Read the model definition and answer for the solid it produces. Units are mm, in the model's axes. A direction names the side the tool comes from. Round coordinates to 2 decimals unless told otherwise and drop trailing zeros. Write each loop counter-clockwise with the first axis right and the second up, starting at its lowest first coordinate (ties: lowest second). Pieces come first, ordered by that corner, then holes.
from build123d import *
from build123d.topology import SkipClean

# Parameters (mm, degrees)
SKETCH_2_R          = 9.25
SKETCH_2_R_2        = 7.25
F_19MM_DEPTH        = 19
EXTRUDE_START       = -11
EXTRUDE_7_DEPTH     = 11
SKETCH_630_W        = 27.57
SKETCH_630_H        = 12
EXTRUDE_682_DEPTH   = 14
SKETCH_6_W          = 25.57
SKETCH_6_H          = 10
CUT_EXTRUDE_1_DEPTH = 12
FILLET_1_R          = 5
SKETCH_10_W         = 27.57
SKETCH_10_H         = 1
EXTRUDE_3_DEPTH     = 8


with BuildPart() as part:
    # 草圖2 → 19mm (new body)
    with BuildSketch(Plane(origin=(0, 0, 0), x_dir=(1, 0, 0), z_dir=(0, 1, 0))):
        Circle(SKETCH_2_R)
        Circle(SKETCH_2_R_2, mode=Mode.SUBTRACT)
    extrude(amount=F_19MM_DEPTH)

    # 草圖14 → 伸長-薄件7 (add)
    with SkipClean():  # the faces are left unmerged after this step: merging them gives an invalid solid
        with BuildSketch(Plane(origin=(0, 0, 0), x_dir=(1, 0, 0), z_dir=(0, 1, 0)).offset(EXTRUDE_START)):
            with BuildLine():
                ThreePointArc((7.25, 0), (0, 7.25), (-7.25, 0))
                Line((-7.25, 0), (-9.25, 0))
                ThreePointArc((-9.25, 0), (0, 9.25), (9.25, 0))
                Line((9.25, 0), (7.25, 0))
            make_face()
        extrude(amount=EXTRUDE_7_DEPTH)

    # Sketch 630 → Extrude 682 (add)
    with SkipClean():  # the faces are left unmerged after this step: merging them gives an invalid solid
        with BuildSketch(Plane.XY):
            with Locations((0, -6)):
                Rectangle(SKETCH_630_W, SKETCH_630_H)
        extrude(amount=EXTRUDE_682_DEPTH)

    # 草圖6 → 除料-伸長1 (cut)
    with SkipClean():  # the faces are left unmerged after this step: merging them gives an invalid solid
        with BuildSketch(Plane.XY.offset(14)):
            with Locations((0, -6)):
                Rectangle(SKETCH_6_W, SKETCH_6_H)
        extrude(amount=-CUT_EXTRUDE_1_DEPTH, mode=Mode.SUBTRACT)

    # 圓角1
    # the kernel refuses this fillet: 5 mm, written as the material it takes off along each edge
    with BuildSketch(Plane(origin=(-19.75, 0, 0), x_dir=(0, -1, 0), z_dir=(1, 0, 0))) as fillet_1_piece_1_section:
        with BuildLine():
            CenterArc((FILLET_1_R, -FILLET_1_R), FILLET_1_R, 90, 90)
            Line((0, -FILLET_1_R), (0, 0))
            Line((0, 0), (FILLET_1_R, 0))
        make_face()
    fillet_1_piece_1 = extrude(amount=39.5, mode=Mode.PRIVATE)
    fillet_1_piece_1 = fillet_1_piece_1 & Plane(origin=(0, -1.958227167, 0), x_dir=(1, 0, 0), z_dir=(0, -1, 0)) * Cylinder(7.25, 99, mode=Mode.PRIVATE)
    add(fillet_1_piece_1, mode=Mode.SUBTRACT)

    # 草圖10 → 填料-伸長3 (add)
    with BuildSketch(Plane.XZ.offset(12)):
        with Locations((0, 0.5)):
            Rectangle(SKETCH_10_W, SKETCH_10_H)
    extrude(amount=EXTRUDE_3_DEPTH)


solid = part.part
Q1. Flat-ended cylindrical pins translate along their axes: pin 1 Ø6.5 at (x, z) = (-0.5, 8.5) entering from -Y; pin 2 Ø1.5 at (y, z) = (-7.5, -7) entering from +X; pin 3 Ø6 at (x, z) = (-1, 4) entering from +Y. Find the tip coordinate at first contact, or state that the pin passes through.
Verdict:
pin 1: stops at y = -12
pin 2: stops at x = 6.82
pin 3: stops at y = 0
Q2. Determine the mould class of faces 1 (the flat face through (0, 0, 10)), 2 (the flat face through (0, -6, 2)), 3 (the cylindrical face through (-0.94, 7.12, -7.19)) for opening direction Y: pulls with the +Y half, pulls with the -Y half, needs draft (parallel to the pull), parting line crosses it, or undercut.
Verdict:
face 1: pulls with the +Y half
face 2: undercut
face 3: needs draft
Q3. Which of the six approach directions +Z, -Z, +X, -X, +Y, -Y give full straight-line access (tool end or side, diameter ignored) to faces 4 (the flat face through (0, -11, 8)), 5 (the flat face through (0, -12, 7)), 6 (the cylindrical face through (-0.098, -0.264, 3.398)), 7 (the flat face through (-0.6, -11, -7.4))?
Verdict:
face 4: +Z
face 5: +Z, +X, -X, -Y
face 6: +Y
face 7: -Z, +X, -X, -Y
Q4. Straight lines are drawn through the part: probe 1 along X at (y, z) = (10.5, 0); probe 2 along X at (y, z) = (-3, 13) (3 decimals); probe 3 along Y at (x, z) = (2.5, 11). For each, find the intervals that lie inside material, in ascending order.
Verdict:
probe 1: x = -9.25 to -7.25, 7.25 to 9.25
probe 2: x = -13.785 to -12.785, 12.785 to 13.785
probe 3: y = -12 to -11, -1 to 0
Q5. Section D-D (x = 11.75) is taken. Determine the outline of the cut face in (y, z).
Verdict:
outline: (-20, 0) - (0, 0) - (0, 14) - (-1, 14) - (-1, 2) - (-11, 2) - (-11, 14) - (-12, 14) - (-12, 1) - (-20, 1) - close
Q6. Section B-B (y = -7.5) is taken. Determine the outline of the cut face in (x, z) (3 decimals).
Verdict:
outline: (-13.785, 0) - (-9.25, 0) arc R9.25 ccw to (9.25, 0) - (13.785, 0) - (13.785, 14) - (12.785, 14) - (12.785, 2) - (-12.785, 2) - (-12.785, 14) - (-13.785, 14) - close; hole (-7.25, 0) arc R7.25 ccw to (7.25, 0) - close
Q7. Section C-C (z = -6.5) is taken. Determine the outline of the cut face in (x, y), then the cut area to 3 significant figures.
Verdict:
outline: (-6.58, -11) - (-3.21, -11) - (-3.21, 19) - (-6.58, 19) - close; (3.21, -11) - (6.58, -11) - (6.58, 19) - (3.21, 19) - close
area: 202 mm2
